Could you check a few things on this model? Use its own coordinates, in mm. Face numbers are marked on the shaded views. A direction names the side the tool comes from. Round coordinates to 2 decimals unless told otherwise and drop trailing zeros. Order: outer loops, then holes, each group sorted by start corner. A loop starts at its lowest first (then second) coordinate and runs counter-clockwise, first axis right, second up.
```python
from build123d import *

# Parameters (mm, degrees)
SKETCH1_W           = 50.8
SKETCH1_H           = 50.8
SKETCH1_W_2         = 44.45
SKETCH1_H_2         = 44.45
BOSS_EXTRUDE1_DEPTH = 300
SKETCH2_R           = 2.5
CUT_EXTRUDE1_DEPTH  = 300


with BuildPart() as part:
    # Sketch1 → Boss-Extrude1 (new body)
    with BuildSketch(Plane(origin=(0, 0, 0), x_dir=(0, 0, -1), z_dir=(1, 0, 0))):
        with Locations((25.4, 25.4)):
            Rectangle(SKETCH1_W, SKETCH1_H)
        with Locations((25.4, 25.4)):
            Rectangle(SKETCH1_W_2, SKETCH1_H_2, mode=Mode.SUBTRACT)
    extrude(amount=BOSS_EXTRUDE1_DEPTH)

    # Sketch2 → Cut-Extrude1 (cut)
    with BuildSketch(Plane.XY):
        with Locations((25.4, 15.875)):
            Circle(SKETCH2_R)
        with Locations((76.2, 15.875)):
            Circle(SKETCH2_R)
        with Locations((127, 15.875)):
            Circle(SKETCH2_R)
        with Locations((177.8, 15.875)):
            Circle(SKETCH2_R)
        with Locations((228.6, 15.875)):
            Circle(SKETCH2_R)
        with Locations((279.4, 15.875)):
            Circle(SKETCH2_R)
        with Locations((76.2, 34.925)):
            Circle(SKETCH2_R)
        with Locations((127, 34.925)):
            Circle(SKETCH2_R)
        with Locations((177.8, 34.925)):
            Circle(SKETCH2_R)
        with Locations((228.6, 34.925)):
            Circle(SKETCH2_R)
        with Locations((279.4, 34.925)):
            Circle(SKETCH2_R)
        with Locations((25.4, 34.925)):
            Circle(SKETCH2_R)
    extrude(amount=-CUT_EXTRUDE1_DEPTH, mode=Mode.SUBTRACT)


solid = part.part
```
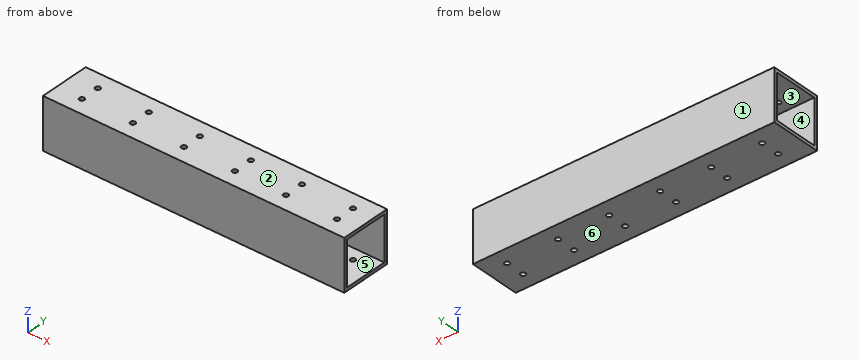
Q1. Imagine slicing it at A-A, the plane x = 228.6. Please give me the cut outline in (y, z) (3 decimals), then the cut area to 3 significant figures.
Q2. For the marked faces 5 and 6, which set-ups out of +Z, -Z, +X, -X, +Y, -Y let a thin tool reach every point of the face, with its end or its side?
Q3. Imagine slicing it at C-C, the plane y = 43. Please give me the cut outline in (x, z) (3 decimals).
Q4. Imagine slicing it at D-D, the plane x = 169. Please give me the cut outline in (y, z) (3 decimals), then the cut area to 3 significant figures.
Q5. I need wall thicknesses on L1, parallel to Y at x = 206, z = -18.5 (3 decimals); L2, parallel to Z at x = 162, y = 22 (3 decimals); L3, parallel to Y at x = 127, z = -0.7 (3 decimals). Which ranges of each line are inside material? Lowest first, please.
Q6. Imagine slicing it at B-B, the plane z = -9.5. Please give me the cut outline in (x, y) (3 decimals).
Q7. We'd pull the mould along Y, two halves only. Please class the marked faces 1, 2, 3 and 4: released by +Y, released by -Y, zero draft, split by the parting line, or undercut.
Q8. For P1, Ø1.5, axis at y = 22.5, z = -45.5, coming from the +X side, with a flat end and sliding along its axis, tell me the tip position at first contact or that it passes through.
Filled in:
1. outline: (0, -50.8) - (13.375, -50.8) - (13.375, -47.625) - (3.175, -47.625) - (3.175, -3.175) - (13.375, -3.175) - (13.375, 0) - (0, 0) - close; (18.375, -50.8) - (32.425, -50.8) - (32.425, -47.625) - (18.375, -47.625) - close; (18.375, -3.175) - (32.425, -3.175) - (32.425, 0) - (18.375, 0) - close; (37.425, -50.8) - (50.8, -50.8) - (50.8, 0) - (37.425, 0) - (37.425, -3.175) - (47.625, -3.175) - (47.625, -47.625) - (37.425, -47.625) - close
1. area: 541 mm2
2. face 5: +X, -X
2. face 6: -Z, +X, -X, +Y, -Y
3. outline: (0, -50.8) - (300, -50.8) - (300, -47.625) - (0, -47.625) - close; (0, -3.175) - (300, -3.175) - (300, 0) - (0, 0) - close
4. outline: (0, -50.8) - (50.8, -50.8) - (50.8, 0) - (0, 0) - close; hole (3.175, -47.625) - (47.625, -47.625) - (47.625, -3.175) - (3.175, -3.175) - close
4. area: 605 mm2
5. L1: y = 0 to 3.175, 47.625 to 50.8
5. L2: z = -50.8 to -47.625, -3.175 to 0
5. L3: y = 0 to 13.375, 18.375 to 32.425, 37.425 to 50.8
6. outline: (0, 0) - (300, 0) - (300, 3.175) - (0, 3.175) - close; (0, 47.625) - (300, 47.625) - (300, 50.8) - (0, 50.8) - close
7. face 1: released by +Y
7. face 2: zero draft
7. face 3: undercut
7. face 4: undercut
8. P1: passes through
